```python
from build123d import *

# Parameters (mm, degrees)
SKETCH1_R                     = 57
EXTRUDE4_DEPTH                = 7.5
EXTRUDE5_DEPTH                = 7.5
EXTRUDE5_DEPTH_BACK           = 5
SKETCH_R                      = 60
SKETCH_R_2                    = 57
SKETCH2_R                     = 14
EXTRUDE6_DEPTH                = 87.168439698
SKETCH6_R                     = 14.8
EXTRUDE7_DEPTH                = 2.5
EXTRUDE8_START                = -16.8000001
EXTRUDE8_OUTLINE_R            = 2
EXTRUDE8_DEPTH                = 2.135757978
EXTRUDE8_START_2              = -3
EXTRUDE8_2_DEPTH              = 6
M8_CLEARANCE_HOLE1_D          = 9
CIRPATTERN1_COUNT             = 4
M5_CLEARANCE_HOLE1_AT_2_COUNT = 2
M5_CLEARANCE_HOLE1_AT_2_PITCH = 36
M5_CLEARANCE_HOLE1_AT_3_COUNT = 2
M5_CLEARANCE_HOLE1_AT_3_PITCH = 83.192547743
M5_CLEARANCE_HOLE1_AT_4_COUNT = 2
M5_CLEARANCE_HOLE1_AT_4_PITCH = 75


with BuildPart() as part:
    # Sketch1 → Extrude4 (new, symmetric)
    with BuildSketch(Plane(origin=(0, 0, 0), x_dir=(1, 0, 0), z_dir=(0, 1, 0))):
        with Locations(Location((0, 0, 0), (0, 0, 270))):
            Circle(SKETCH1_R)
    extrude(amount=EXTRUDE4_DEPTH, both=True)

    # Sketch → Extrude5 (add, two sides: drawn at the far end of the back side and taken through both)
    with BuildSketch(Plane(origin=(0, 0, 0), x_dir=(1, 0, 0), z_dir=(0, 1, 0)).offset(-EXTRUDE5_DEPTH_BACK)):
        with Locations(Location((0, 0, 0), (0, 0, 270))):
            Circle(SKETCH_R)
        with Locations(Location((0, 0, 0), (0, 0, 270))):
            Circle(SKETCH_R_2, mode=Mode.SUBTRACT)
    extrude(amount=EXTRUDE5_DEPTH + EXTRUDE5_DEPTH_BACK)

    # Sketch2 → Extrude6 (cut, through all)
    with BuildSketch(Plane(origin=(0, 7.5, 0), x_dir=(1, 0, 0), z_dir=(0, 1, 0))):
        with Locations(Location((0, 0, 0), (0, 0, 270))):
            Circle(SKETCH2_R)
    extrude(amount=-EXTRUDE6_DEPTH, mode=Mode.SUBTRACT)

    # Sketch6 → Extrude7 (cut, symmetric)
    with BuildSketch(Plane(origin=(0, 0, 0), x_dir=(1, 0, 0), z_dir=(0, 1, 0))):
        with Locations(Location((0, 0, 0), (0, 0, 270))):
            Circle(SKETCH6_R)
    extrude(amount=EXTRUDE7_DEPTH, both=True, mode=Mode.SUBTRACT)

    # Extrude8: read off the stored shape, not the designer's step
    # Extrude8 outline → Extrude8 (cut)
    with BuildSketch(Plane.XY.offset(EXTRUDE8_START)):
        Circle(EXTRUDE8_OUTLINE_R)
    extrude(amount=EXTRUDE8_DEPTH, mode=Mode.SUBTRACT)

    # Extrude8 2 outline → Extrude8 2 (add)
    with BuildSketch(Plane(origin=(0, 0, 0), x_dir=(1, 0, 0), z_dir=(0, 1, 0)).offset(EXTRUDE8_START_2)):
        with BuildLine():
            ThreePointArc((-2e-09, 16.8), (1.002059984, 16.770088723), (2.000551768, 16.680461403))
            Line((2.000551768, 16.680461403), (3, 16.56059374))
            Line((3, 16.56059374), (3, 16.8000001))
            Line((3, 16.8000001), (-2e-09, 16.8))
        make_face()
        with BuildLine():
            ThreePointArc((-2.000001192, 16.680527427), (-1.001783219, 16.770105259), (-2e-09, 16.8))
            Line((-2e-09, 16.8), (-3, 16.8000001))
            Line((-3, 16.8000001), (-3, 16.560627213))
            Line((-3, 16.560627213), (-2.000001192, 16.680527427))
        make_face()
    extrude(amount=EXTRUDE8_2_DEPTH)

    # M8 Clearance Hole1 (through all)
    with Locations(Plane(origin=(0, 7.5, 0), x_dir=(1, 0, 0), z_dir=(0, 1, 0))):
        with Locations((-35.355339059, -35.355339059)):
            m8_clearance_hole1 = Hole(M8_CLEARANCE_HOLE1_D / 2)

    # CirPattern1: M8 Clearance Hole1 ×4 about axis
    cirpattern1_axis = Axis((0, 0, 0), (0, 1, 0))
    for i in range(1, CIRPATTERN1_COUNT):
        add(m8_clearance_hole1.rotate(cirpattern1_axis, i * 360 / CIRPATTERN1_COUNT), mode=Mode.SUBTRACT)

    # Sketch10 → M5 Clearance Hole1 (revolve, cut)
    with BuildSketch(Plane(origin=(37.5, -7.5, 18), x_dir=(0, 0, -1), z_dir=(1, 0, 0))):
        Polygon((0, 0), (0, 15), (4.7, 15), (2.75, 13.05), (2.75, 0), align=None)
    m5_clearance_hole1 = revolve(axis=Axis((37.5, -13.85, 18), (0, 1, 0)), mode=Mode.SUBTRACT)

    # M5 Clearance Hole1 at 2: M5 Clearance Hole1 ×2
    with Locations(*[(0, 0, -i * M5_CLEARANCE_HOLE1_AT_2_PITCH) for i in range(1, M5_CLEARANCE_HOLE1_AT_2_COUNT)]):
        add(m5_clearance_hole1, mode=Mode.SUBTRACT)

    # M5 Clearance Hole1 at 3: M5 Clearance Hole1 ×2
    with Locations(*[Vector(-0.9015230574682735, 0, -0.4327310675847715) * (i * M5_CLEARANCE_HOLE1_AT_3_PITCH) for i in range(1, M5_CLEARANCE_HOLE1_AT_3_COUNT)]):
        add(m5_clearance_hole1, mode=Mode.SUBTRACT)

    # M5 Clearance Hole1 at 4: M5 Clearance Hole1 ×2
    with Locations(*[(-i * M5_CLEARANCE_HOLE1_AT_4_PITCH, 0, 0) for i in range(1, M5_CLEARANCE_HOLE1_AT_4_COUNT)]):
        add(m5_clearance_hole1, mode=Mode.SUBTRACT)


solid = part.part
```
Source: CAD feature listing. Evaluate the final solid. Frame: model axes, mm. A direction names the side the tool comes from. Give positions to 0.01 mm unless a question says otherwise; leave off trailing zeros. Write each loop counter-clockwise with the first axis right and the second up, starting at its lowest first coordinate (ties: lowest second). Pieces come first, ordered by that corner, then holes. Notation, with made-up numbers: (-30, 27) - (7, 27) arc R5 cw to (7, 31) - close; hole circle Ø2 at (-12.5, 43). An arc over 180 degrees is marked (long way). One line per item, written item: value. Start each with the question number.
Q1. Section query B-B, the plane z = -33. Return the cut outline in (x, y), then the cut area to 3 significant figures.
Q2. Section query C-C, the plane z = -6. Return the cut outline in (x, y), then the cut area to 3 significant figures.
Q3. Draft query along Z for faces 4 (the face through (2.64, 1.16, -59.94)), 5 (the face through (14.2, 7.5, -0.8)), 6 (the face through (34.773, -1.066, 18.358)). Return one class per face: +Z half, -Z half, draft (parallel to the pull), parting line (faces both ways), or undercut.
Q4. Material intervals for probe 1 along X at (y, z) = (3.25, 35); probe 2 along X at (y, z) = (6, 0.5); probe 3 along Z at (x, y) = (-38, -6.5), sorted ascending. Write a range as from..to.
Q5. Section query D-D, the plane x = -53. Return the cut outline in (y, z).
Q6. Section query A-A, the plane x = -37.5. Return the cut outline in (y, z).
Q7. Set-up query: faces 1 (the face through (-40.227, -1.066, 18.358)), 2 (the face through (-22, -5, 53)), 3 (the face through (-5.67, 0.04, 13.67)). Return all of +Z, -Z, +X, -X, +Y, -Y with unobstructed straight access to the full face (end or side cutting, diameter ignored); none if empty.
Q8. First-contact query: pin 1 Ø6 at (y, z) = (1.5, 40) entering from +X; pin 2 Ø6 at (x, y) = (-6, -2.5) entering from -Z; pin 3 Ø3 at (y, z) = (1, -20.5) entering from +X. Flat tips, straight axial feed; report the tip coordinate or a pass-through.
Answer:
1. outline: (-50.11, -5) - (-46.48, -5) - (-46.48, -7.5) - (-39.19, -7.5) - (-39.19, 7.5) - (-50.11, 7.5) - close; (-31.52, -7.5) - (31.52, -7.5) - (31.52, 7.5) - (-31.52, 7.5) - close; (39.19, -7.5) - (46.48, -7.5) - (46.48, -5) - (50.11, -5) - (50.11, 7.5) - (39.19, 7.5) - close
1. area: 1,260 mm2
2. outline: (-59.7, -5) - (-56.68, -5) - (-56.68, -7.5) - (-12.65, -7.5) - (-12.65, -2.5) - (-13.53, -2.5) - (-13.53, 2.5) - (-12.65, 2.5) - (-12.65, 7.5) - (-59.7, 7.5) - close; (12.65, -7.5) - (56.68, -7.5) - (56.68, -5) - (59.7, -5) - (59.7, 7.5) - (12.65, 7.5) - (12.65, 2.5) - (13.53, 2.5) - (13.53, -2.5) - (12.65, -2.5) - close
2. area: 1,390 mm2
3. face 4: parting line
3. face 5: draft
3. face 6: undercut
4. probe 1: x = -48.73..-39.84, -30.87..30.87, 39.84..48.73
4. probe 2: x = -60..-13.99, 13.99..60
4. probe 3: z = -42.49..-39, -31.71..-20.7, -15.3..15.3, 20.7..31.71, 39..42.49
5. outline: (-7.5, -20.98) - (-5, -20.98) - (-5, -28.12) - (7.5, -28.12) - (7.5, 28.12) - (-5, 28.12) - (-5, 20.98) - (-7.5, 20.98) - close
6. outline: (-7.5, -42.93) - (-5, -42.93) - (-5, -46.84) - (7.5, -46.84) - (7.5, -39.31) - (-7.5, -39.31) - close; (-7.5, -31.4) - (7.5, -31.4) - (7.5, -22.7) - (5.55, -20.75) - (-7.5, -20.75) - close; (-7.5, -15.25) - (5.55, -15.25) - (7.5, -13.3) - (7.5, 13.3) - (5.55, 15.25) - (-7.5, 15.25) - close; (-7.5, 20.75) - (5.55, 20.75) - (7.5, 22.7) - (7.5, 31.4) - (-7.5, 31.4) - close; (-7.5, 39.31) - (7.5, 39.31) - (7.5, 46.84) - (-5, 46.84) - (-5, 42.93) - (-7.5, 42.93) - close
7. face 1: +Y, -Y
7. face 2: -Y
7. face 3: none
8. pin 1: stops at x = 47.23
8. pin 2: stops at z = -59.92
8. pin 3: stops at x = 56.91
